from build123d import *

# Parameters (mm, degrees)
F0_W     = 80
F0_H     = 60
F1_DEPTH = 40
F2_W     = 80
F2_H     = 10
F3_DEPTH = 2
F5_DEPTH = 2
F7_DEPTH = 2
F9_DEPTH = 2


with BuildPart() as f1:
    # F0 (on Top) → F1 (new body)
    with BuildSketch(Plane.XY):
        Rectangle(F0_W, F0_H)
    extrude(amount=F1_DEPTH)

    # F2 (on face) → F3 (join)
    with BuildSketch(Plane.XZ.offset(30)):
        with Locations((0, 35)):
            Rectangle(F2_W, F2_H)
    extrude(amount=F3_DEPTH)

    # F4 (on face) → F5 (join)
    with BuildSketch(Plane.YZ.offset(40)):
        Polygon((-32, 40), (-32, 30), (-30, 30), (30, 30), (30, 40), align=None)
    extrude(amount=F5_DEPTH)

    # F6 (on face) → F7 (join)
    with BuildSketch(Plane(origin=(0, 30, 0), x_dir=(-1, 0, 0), z_dir=(0, 1, 0))):
        Polygon((-42, 40), (-42, 30), (-40, 30), (40, 30), (40, 40), align=None)
    extrude(amount=F7_DEPTH)

    # F8 (on face) → F9 (join)
    with BuildSketch(Plane(origin=(-40, 0, 0), x_dir=(0, -1, 0), z_dir=(-1, 0, 0))):
        Polygon((-32, 40), (-32, 30), (-30, 30), (30, 30), (32, 30), (32, 40), align=None)
    extrude(amount=F9_DEPTH)


solid = f1.part
Could you check a few things on this model? Use its own coordinates, in mm. A direction names the side the tool comes from. Coordinates: 2 decimals unless noted, no trailing zeros. Write each loop counter-clockwise with the first axis right and the second up, starting at its lowest first coordinate (ties: lowest second). Pieces come first, ordered by that corner, then holes. Notation, with made-up numbers: (47.25, 8) - (90.25, 8) arc R7 ccw to (90.25, 16) - close; hole circle Ø10 at (-38, 23). An arc over 180 degrees is marked (long way). Put each result on its own line as item: value. Start each with the question number.
Q1. I want a section at C-C on z = 28.5. Write out the boundary of the cut face in (x, y), plus the area to 3 significant figures.
Q2. I want a section at B-B on y = 23.5. Write out the boundary of the cut face in (x, z).
Q3. I want a section at A-A on x = 35.5. Write out the boundary of the cut face in (y, z).
Q4. Please list where these lines run through material, in increasing order: L1, parallel to Y at x = -33, z = 17; L2, parallel to X at y = 22.5, z = 7.5.
Q5. I'm going to push flat-ended pins straight in: P1, Ø4, axis at x = -14.5, z = 12.5, coming from the +Y side; P2, Ø15, axis at y = -14.5, z = 11.5, coming from the +X side; P3, Ø15, axis at x = -13.5, z = 16.5, coming from the -Y side. Where does each tip first touch, or does it pass through?
Q6. Which directions (+Z, -Z, +X, -X, +Y, -Y) give clear straight access to the entire face, cutting with the end or side of a thin tool? Please do faces 1 (the flat face through (-1, -30, 15)), 2 (the flat face through (-40, 0, 15)), 3 (the flat face through (-1, 30, 15)).
Checks:
1. outline: (-40, -30) - (40, -30) - (40, 30) - (-40, 30) - close
1. area: 4,800 mm²
2. outline: (-42, 30) - (-40, 30) - (-40, 0) - (40, 0) - (40, 30) - (42, 30) - (42, 40) - (-42, 40) - close
3. outline: (-32, 30) - (-30, 30) - (-30, 0) - (30, 0) - (30, 30) - (32, 30) - (32, 40) - (-32, 40) - close
4. L1: -30 to 30
4. L2: -40 to 40
5. P1: y = 30
5. P2: x = 40
5. P3: y = -30
6. face 1: -Z, +X, -X, -Y
6. face 2: -Z, -X, +Y, -Y
6. face 3: -Z, +X, -X, +Y
